Can you work these out from the model? Positions are in its coordinate system, mm. Face numbers are marked on the shaded views. A direction names the side the tool comes from. Coordinates: 2 decimals unless noted, no trailing zeros. Loops run counter-clockwise (first coordinate to the right, second up) from the corner with the lowest first, then second, coordinate; pieces in that order, holes last. Notation, with made-up numbers: M -39,38.5 L -12,38.5 A22 ccw -12,70.5 Z; hole C -6,41.25 d3. An arc over 180 degrees is marked long. Answer as a JSON object with one key per item and string values. Group by question number.
Item 1: Suppose I cut it at A-A (z = 572). Write out the boundary of the cut face in (x, y).
Item 2: Suppose I cut it at B-B (x = 25). Write out the boundary of the cut face in (y, z).
Item 3: Which directions (+Z, -Z, +X, -X, +Y, -Y) give clear straight access to the entire face, cutting with the end or side of a thin tool? Please do the marked faces 1 and 2.
Item 4: If I drill on line 1 (Y direction, x = 48, z = 109); line 2 (X direction, y = -34.5, z = 418); line 3 (Y direction, x = 9.5, z = 475.5), over which ranges is the centre line in solid material (lowest first)?
Item 5: I'm going to push flat-ended pins straight in: pin 1 Ø10 at (x, z) = (19.5, 189) entering from -Y; pin 2 Ø5.5 at (y, z) = (-20.066, 109.22) entering from -X; pin 3 Ø8.5 at (y, z) = (-20.066, 109.22) entering from -X; pin 4 Ø2.5 at (x, y) = (12.5, -1.5) entering from -Z. Where does each tip first touch, or does it pass through?
```python
from build123d import *

# Parameters (mm, degrees)
BOSS_EXTRUDE1_DEPTH = 609.6
SKETCH3_W           = 92.456
SKETCH3_H           = 123.444
CUT_EXTRUDE1_DEPTH  = 614.028039672
SKETCH4_R           = 3.175
CUT_EXTRUDE2_DEPTH  = 620.310340156


with BuildPart() as part:
    # Sketch1 → Boss-Extrude1 (new body)
    with BuildSketch(Plane.XY):
        Polygon((-50.8, 0), (50.8, 0), (50.8, -40.132), (46.228, -40.132), (46.228, -4.572), (-46.228, -4.572), (-46.228, -40.132), (-50.8, -40.132), align=None)
    extrude(amount=BOSS_EXTRUDE1_DEPTH)

    # Sketch3 → Cut-Extrude1 (cut, through all)
    with BuildSketch(Plane(origin=(0, 0, 0), x_dir=(1, 0, 0), z_dir=(0, 1, 0))):
        with Locations((0, -61.722)):
            Rectangle(SKETCH3_W, SKETCH3_H)
    extrude(amount=-CUT_EXTRUDE1_DEPTH, mode=Mode.SUBTRACT)

    # Sketch4 → Cut-Extrude2 (cut, through all)
    with BuildSketch(Plane(origin=(50.8, 0, 0), x_dir=(0, 0, -1), z_dir=(1, 0, 0))):
        with Locations(Location((-109.22, -20.066, 0), (0, 0, 90))):
            Circle(SKETCH4_R)
        with BuildLine():
            Line((-12.7, -24.8285), (-22.86, -24.8285))
            ThreePointArc((-22.86, -24.8285), (-27.6225, -20.066), (-22.86, -15.3035))
            Line((-22.86, -15.3035), (-12.7, -15.3035))
            ThreePointArc((-12.7, -15.3035), (-7.9375, -20.066), (-12.7, -24.8285))
        make_face()
    extrude(amount=-CUT_EXTRUDE2_DEPTH, mode=Mode.SUBTRACT)


solid = part.part
```
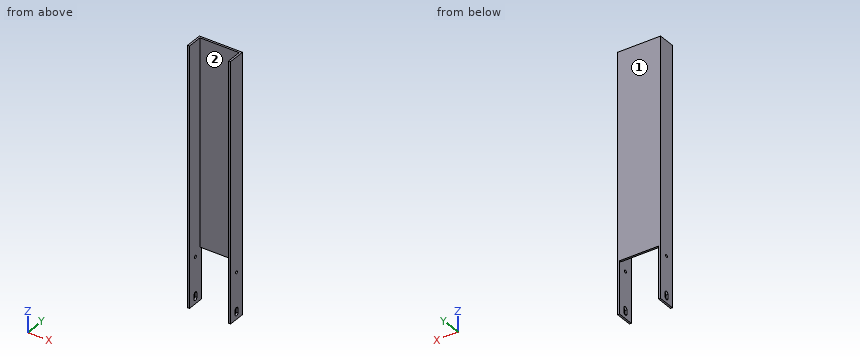
From the geometry:
{
 "1": {"outline": "M -50.8,-40.13 L -46.23,-40.13 L -46.23,-4.57 L 46.23,-4.57 L 46.23,-40.13 L 50.8,-40.13 L 50.8,0 L -50.8,0 Z"},
 "2": {"outline": "M -4.57,123.44 L 0,123.44 L 0,609.6 L -4.57,609.6 Z"},
 "3": {"face 1": "+Z, -Z, +X, -X, +Y", "face 2": "+Z, -Z, -Y"},
 "4": {"line 1": "-40.13 to -23.23, -16.9 to 0", "line 2": "-50.8 to -46.23, 46.23 to 50.8", "line 3": "-4.57 to 0"},
 "5": {"pin 1": "y = -4.57", "pin 2": "through", "pin 3": "x = -50.8", "pin 4": "z = 123.44"}
}
